Read the model definition and answer for the solid it produces. Units are mm, in the model's axes. A direction names the side the tool comes from. Round coordinates to 2 decimals unless told otherwise and drop trailing zeros. Loops run counter-clockwise (first coordinate to the right, second up) from the corner with the lowest first, then second, coordinate; pieces in that order, holes last. Notation, with made-up numbers: (7.25, 29) - (21.25, 29) arc R30 cw to (21.25, 57) - close; hole circle Ø4 at (78, 82). An arc over 180 degrees is marked (long way). Use CSV: the item, a comma, the result in double quotes. Start each with the question number.
1. Find section A-A (x = 0). Give the vertices of the cut face in (y, z).
2. A tool of negligible diameter and unlimited length cuts with its end or side. For faces 1 (the flat face through (-4.545, -4.257, 1.479)), 2 (the cylindrical face through (-0.2, 2.5, 1.5)), 3 (the cylindrical face through (-7.22, -6.125, 1.479)), from which of +Z, -Z, +X, -X, +Y, -Y can it reach the whole face along a straight path? Write none if from no direction.
3. Consider line 1 along X through (y, z) = (-0.25, 2.4); line 2 along X through (y, z) = (-0.75, 0.4); line 3 along X through (y, z) = (-3, 2.55). Determine where each line is inside the solid, lowest interval first.
4. Find section D-D (x = -5). Give the vertices of the cut face in (y, z).
5. Determine the mould class of faces 4 (the flat face through (0, -2, 3)), 5 (the cylindrical face through (-12.2, 0.36, 1.48)), 6 (the cylindrical face through (7.25, -0.77, 1.48)) for opening direction X: +X half, -X half, draft (parallel to the pull), parting line (faces both ways), or undercut.
6. Find section C-C (z = 1.45). Give the vertices of the cut face in (x, y), and give its area (3 significant figures).
7. Given pin 1 Ø1.5 at (x, z) = (3.5, 2) entering from -Y; pin 2 Ø1.2 at (x, y) = (0, 0) entering from -Z, each flat-ended and moving along its own axis, determine where each tip first touches the part or whether it passes through.
8. Find section B-B (y = 0). Give the vertices of the cut face in (x, z), and give its area (3 significant figures).
Autodesk Inventor part; units mm, degrees
ref_plane "YZ Plane" through (0, 0, 0) normal (1, 0, 0) x (0, 1, 0)
ref_plane "XZ Plane" through (0, 0, 0) normal (0, 1, 0) x (-1, 0, 0)
ref_plane "XY Plane" through (0, 0, 0) normal (0, 0, 1) x (1, 0, 0)
sketch "Sketch1" plane through (0, 0, 0) normal (0, 0, 1) x (1, 0, 0)
  circle A0 centre (0, 0) radius 1
  arc A1 (10.9174, 1.2936) -> (-10.9174, 1.2936) centre (0, -47.5) ccw
  line L0 (-11.3763, -5.0432) -> (-12.4125, -1.1758)
  line L1 (0, -47.5) -> (0, 2.5) construction
  line L2 (11.3763, -5.0432) -> (12.4125, -1.1758)
  line L3 (-10.8704, -6.9311) -> (0, -47.5) construction
  line L4 (-4.4935, -4.7471) -> (-4.5981, -3.7523)
  line L5 (4.4935, -4.7471) -> (4.5981, -3.7523)
  arc A2 (9.0151, -6.4789) -> (5.3604, -5.8435) centre (0, -47.5) ccw
  arc A3 (-5.3604, -5.8435) -> (-9.0151, -6.4789) centre (0, -47.5) ccw
  line L6 (0, -47.5) -> (-4.3902, -5.7301) construction
  arc A4 (3.6854, -2.6512) -> (-3.6854, -2.6512) centre (0, -47.5) ccw
  circle A5 centre (0, -47.5) radius 47.5 construction
  circle A6 centre (8.2483, -0.7216) radius 1
  circle A7 centre (-8.2483, -0.7216) radius 1
  line L7 (0, -47.5) -> (-8.2483, -0.7216) construction
  arc A8 (-10.9174, 1.2936) -> (-12.4125, -1.1758) centre (-10.4807, -0.6582) ccw
  arc A9 (-11.3763, -5.0432) -> (-9.0151, -6.4789) centre (-9.4444, -4.5256) ccw
  arc A10 (12.4125, -1.1758) -> (10.9174, 1.2936) centre (10.4807, -0.6582) ccw
  arc A11 (9.0151, -6.4789) -> (11.3763, -5.0432) centre (9.4444, -4.5256) ccw
  arc A12 (-3.6854, -2.6512) -> (-4.5981, -3.7523) centre (-3.6035, -3.6478) ccw
  arc A13 (4.5981, -3.7523) -> (3.6854, -2.6512) centre (3.6035, -3.6478) ccw
  arc A14 (4.4935, -4.7471) -> (5.3604, -5.8435) centre (5.488, -4.8517) ccw
  arc A15 (-5.3604, -5.8435) -> (-4.4935, -4.7471) centre (-5.488, -4.8517) ccw
  point P0 (-12.941, 0.7963)
  point P1 (12.941, 0.7963)
  point P2 (-10.8704, -6.9311)
  point P3 (10.8704, -6.9311)
  point P4 (-4.7038, -2.7465)
  point P5 (4.7038, -2.7465)
  point P6 (-4.3902, -5.7301)
  point P7 (4.3902, -5.7301)
  dimension "d0" = 2
  dimension "d1" = 100
  dimension "d2" = 47.5
  dimension "d4" = 30
  dimension "d5" = 15
  dimension "d7" = 12
  dimension "d8" = 42
  dimension "d9" = 45
  dimension "d10" = 2
  dimension "d11" = 10
  dimension "d12" = 2
  dimension "d13" = 1
extrude "Extrusion1" add sketch "Sketch1" along normal blind 3
properties part number "bump_sensor_mount"
Filled sheet:
1,outline,"(-2.5, 0) - (-1, 0) - (-1, 3) - (-2.5, 3) - close; (1, 0) - (2.5, 0) - (2.5, 3) - (1, 3) - close"
2,face 1,"+Z, -Z"
2,face 2,"+Z, -Z, +Y"
2,face 3,"+Z, -Z, -Y"
3,line 1,"x = -12.44 to -9.13, -7.37 to -0.97, 0.97 to 7.37, 9.13 to 12.44"
3,line 2,"x = -12.48 to -9.25, -7.25 to -0.66, 0.66 to 7.25, 9.25 to 12.48"
3,line 3,"x = -11.92 to -4.37, 4.37 to 11.92"
4,outline,"(-5.72, 0) - (2.25, 0) - (2.25, 3) - (-5.72, 3) - close"
5,face 4,"draft"
5,face 5,"-X half"
5,face 6,"undercut"
6,outline,"(-12.41, -1.18) - (-11.38, -5.04) arc R2 ccw to (-9.02, -6.48) arc R42.03 cw to (-5.36, -5.84) arc R1 ccw to (-4.49, -4.75) - (-4.6, -3.75) arc R1 cw to (-3.69, -2.65) arc R45 cw to (3.69, -2.65) arc R1 cw to (4.6, -3.75) - (4.49, -4.75) arc R1 ccw to (5.36, -5.84) arc R41.97 cw to (9.02, -6.48) arc R2 ccw to (11.38, -5.04) - (12.41, -1.18) arc R2 ccw to (10.92, 1.29) arc R50 ccw to (-10.92, 1.29) arc R2 ccw to start; hole circle Ø2 at (-8.25, -0.72); hole circle Ø2 at (0, 0); hole circle Ø2 at (8.25, -0.72)"
6,area,"153 mm²"
7,pin 1,"stops at y = -2.88"
7,pin 2,"passes through"
8,outline,"(-12.37, 0) - (-8.94, 0) - (-8.94, 3) - (-12.37, 3) - close; (-7.56, 0) - (-1, 0) - (-1, 3) - (-7.56, 3) - close; (1, 0) - (7.56, 0) - (7.56, 3) - (1, 3) - close; (8.94, 0) - (12.37, 0) - (12.37, 3) - (8.94, 3) - close"
8,area,"59.9 mm²"
